from build123d import *

# Parameters (mm, degrees)
F0_W     = 66.4
F0_H     = 55
F0_W_2   = 49
F0_H_2   = 47.5
F1_DEPTH = 21
F2_DEPTH = 41.5
F3_R     = 1


with BuildPart() as f1:
    # F0 (on Top) → F1 (new body)
    with BuildSketch(Plane.XY):
        Rectangle(F0_W, F0_H)
        Rectangle(F0_W_2, F0_H_2, mode=Mode.SUBTRACT)
    extrude(amount=F1_DEPTH)

    # F0 (on Top) → F2 (join)
    with BuildSketch(Plane.XY):
        Rectangle(F0_W_2, F0_H_2)
    extrude(amount=F2_DEPTH)

    # F3
    f3_edges = [f1.edges().sort_by_distance(p)[0] for p in [
        (0, 23.75, 41.5),
        (-24.5, 0, 41.5),
        (0, -23.75, 41.5),
        (24.5, 0, 41.5),
        (-24.5, 0, 21),
        (-24.5, -23.75, 31.25),
        (-24.5, 23.75, 31.25),
        (0, -23.75, 21),
        (24.5, -23.75, 31.25),
        (33.2, -27.5, 10.5),
        (33.2, 27.5, 10.5),
        (33.2, 0, 0),
        (33.2, 0, 21),
        (-33.2, -27.5, 10.5),
        (0, -27.5, 0),
        (0, -27.5, 21),
        (-33.2, 27.5, 10.5),
        (-33.2, 0, 0),
        (-33.2, 0, 21),
        (0, 27.5, 0),
        (0, 27.5, 21),
        (24.5, 0, 21),
        (0, 23.75, 21),
    ]]
    fillet(f3_edges, radius=F3_R)


solid = f1.part
Geometry: final body of the model. Coordinates: model frame, mm. A direction names the side the tool comes from. Give positions to 0.01 mm unless a question says otherwise; leave off trailing zeros. Write each loop counter-clockwise with the first axis right and the second up, starting at its lowest first coordinate (ties: lowest second). Pieces come first, ordered by that corner, then holes.
(1) First-contact query: P1, Ø5.5, axis at x = -1.5, z = 28, coming from the +Y side; P2, Ø9, axis at y = 9, z = 35.5, coming from the -X side; P3, Ø5.5, axis at y = -1.5, z = 29.5, coming from the +X side. Flat tips, straight axial feed; report the tip coordinate or a pass-through.
(2) Cut plane B-B, the plane z = 33.5. Return loops of the section in (x, y).
(3) Cut plane A-A, the plane x = 0.5. Return loops of the section in (y, z).
(4) Cut plane C-C, the plane y = 15. Return loops of the section in (x, z).
(5) Ray query, line 1 (Z direction, x = -29, y = -22); line 2 (Y direction, x = -15, z = 39); line 3 (X direction, y = 9, z = 30.5). Return the intervals inside material, ascending.
(6) Access query for faces 1 (the flat face through (0, 23.75, 31)), 2 (the flat face through (-24.5, 0, 31)), 3 (the flat face through (0, -23.75, 31)), 4 (the flat face through (24.5, 0, 31)). Directions: +Z, -Z, +X, -X, +Y, -Y. A direction counts if a zero-diameter tool reaches every point of the face in a straight line with its end or side. Return the directions, or none.
Values follow:
1. P1: stops at y = 23.75
1. P2: stops at x = -24.5
1. P3: stops at x = 24.5
2. outline: (-24.5, -22.75) arc R1 ccw to (-23.5, -23.75) - (23.5, -23.75) arc R1 ccw to (24.5, -22.75) - (24.5, 23.75) - (-23.5, 23.75) arc R1 ccw to (-24.5, 22.75) - close
3. outline: (-27.5, 1) arc R1 ccw to (-26.5, 0) - (26.5, 0) arc R1 ccw to (27.5, 1) - (27.5, 20) arc R1 ccw to (26.5, 21) - (24.75, 21) arc R1 cw to (23.75, 22) - (23.75, 40.5) arc R1 ccw to (22.75, 41.5) - (-22.75, 41.5) arc R1 ccw to (-23.75, 40.5) - (-23.75, 22) arc R1 cw to (-24.75, 21) - (-26.5, 21) arc R1 ccw to (-27.5, 20) - close
4. outline: (-33.2, 1) arc R1 ccw to (-32.2, 0) - (32.2, 0) arc R1 ccw to (33.2, 1) - (33.2, 20) arc R1 ccw to (32.2, 21) - (25.5, 21) arc R1 cw to (24.5, 22) - (24.5, 40.5) arc R1 ccw to (23.5, 41.5) - (-23.5, 41.5) arc R1 ccw to (-24.5, 40.5) - (-24.5, 22) arc R1 cw to (-25.5, 21) - (-32.2, 21) arc R1 ccw to (-33.2, 20) - close
5. line 1: z = 0 to 21
5. line 2: y = -23.75 to 23.75
5. line 3: x = -24.5 to 24.5
6. face 1: +Z, +X, -X, +Y
6. face 2: +Z, -X, +Y, -Y
6. face 3: +Z, +X, -X, -Y
6. face 4: +Z, +X, +Y, -Y
